```python
from build123d import *

# Parameters (mm, degrees)
BOSS_EXTRUDE1_DEPTH = 5
SKETCH2_R           = 8
BOSS_EXTRUDE2_DEPTH = 25
CHAMFER1_SIZE       = 1


with BuildPart() as part:
    # Sketch1 → Boss-Extrude1 (new body)
    with BuildSketch(Plane(origin=(0, 0, 0), x_dir=(1, 0, 0), z_dir=(0, 1, 0))):
        Polygon((9.517177276, -5.454967463), (9.482729038, 5.514633562), (-0.034448238, 10.969601025), (-9.517177276, 5.454967463), (-9.482729038, -5.514633562), (0.034448238, -10.969601025), align=None)
    extrude(amount=BOSS_EXTRUDE1_DEPTH)

    # Sketch2 → Boss-Extrude2 (add)
    with BuildSketch(Plane(origin=(0, 0, 0), x_dir=(1, 0, 0), z_dir=(0, 1, 0))):
        Circle(SKETCH2_R)
    extrude(amount=BOSS_EXTRUDE2_DEPTH)

    # Chamfer1
    chamfer1_edges = [part.edges().sort_by_distance(p)[0] for p in [
        (-8, 25, 0),
    ]]
    chamfer(chamfer1_edges, length=CHAMFER1_SIZE)


solid = part.part
```
Geometry check sheet. Reference: the model listing, model coordinates, mm. A direction names the side the tool comes from. Coordinates: 2 decimals unless noted, no trailing zeros. Loops run counter-clockwise (first coordinate to the right, second up) from the corner with the lowest first, then second, coordinate; pieces in that order, holes last. Notation, with made-up numbers: (52.5, 33) - (103.5, 33) arc R25 ccw to (103.5, 45) - close; hole circle Ø5 at (23.5, 7). An arc over 180 degrees is marked (long way). One line per item, written item: value. Start each with the question number.
(1) Material ranges on line 1 (X direction, y = 3.25, z = -3); line 2 (Y direction, x = -0.75, z = 9.25); line 3 (X direction, y = 16, z = 1.5), recorded low to high. Write a range as [from, to].
(2) Tool access check on faces 1 (the flat face through (-4.71, 2.46, -8.25)), 2 (the flat face through (-6, 5, 6)). Record the directions out of +Z, -Z, +X, -X, +Y, -Y that give a thin tool (end or side, any length) a straight path to the whole face; none if there is none.
(3) Depth check by flat-ended pin: P1, Ø1.5, axis at y = 19, z = -3, coming from the +X side; P2, Ø5, axis at y = 16.5, z = 2.5, coming from the +X side; P3, Ø1, axis at y = 6.5, z = -2.5, coming from the -X side. Enter the tip coordinate at first touch or a pass-through.
(4) Cross-section at A-A on z = 0. Enter the section's corners in (x, y).
(5) Cross-section at B-B on y = 21.25. Enter the section's corners in (x, z), plus the area to 3 significant figures.
Results below:
1. line 1: x = [-9.51, 9.49]
1. line 2: y = [0, 5]
1. line 3: x = [-7.86, 7.86]
2. face 1: -Z, -X, +Y, -Y
2. face 2: +Y
3. P1: stops at x = 7.68
3. P2: stops at x = 8
3. P3: stops at x = -7.75
4. outline: (-9.5, 0) - (9.5, 0) - (9.5, 5) - (8, 5) - (8, 24) - (7, 25) - (-7, 25) - (-8, 24) - (-8, 5) - (-9.5, 5) - close
5. outline: circle Ø16 at (0, 0)
5. area: 201 mm2
